from build123d import *

# Parameters (mm, degrees)
SKETCH1_R           = 4
SKETCH1_R_2         = 2
BOSS_EXTRUDE1_DEPTH = 5.4
SKETCH2_R           = 7.5
SKETCH2_R_2         = 4
BOSS_EXTRUDE2_DEPTH = 19


with BuildPart() as part:
    # Sketch1 → Boss-Extrude1 (new body)
    with BuildSketch(Plane(origin=(0, 0, 0), x_dir=(0, 0, -1), z_dir=(1, 0, 0))):
        Polygon((-12.5, 10), (-10, 12.5), (10, 12.5), (12.5, 10), (12.5, -10), (10, -12.5), (-10, -12.5), (-12.5, -10), align=None)
        with Locations(Location((0, 0, 0), (0, 0, 180))):
            Circle(SKETCH1_R, mode=Mode.SUBTRACT)
        with Locations(Location((8.485281374, 8.485281374, 0), (0, 0, 180))):
            Circle(SKETCH1_R_2, mode=Mode.SUBTRACT)
        with Locations(Location((8.485281374, -8.485281374, 0), (0, 0, 180))):
            Circle(SKETCH1_R_2, mode=Mode.SUBTRACT)
        with Locations(Location((-8.485281374, -8.485281374, 0), (0, 0, 180))):
            Circle(SKETCH1_R_2, mode=Mode.SUBTRACT)
        with Locations(Location((-8.485281374, 8.485281374, 0), (0, 0, 180))):
            Circle(SKETCH1_R_2, mode=Mode.SUBTRACT)
    extrude(amount=BOSS_EXTRUDE1_DEPTH)

    # Sketch2 → Boss-Extrude2 (add)
    with BuildSketch(Plane(origin=(5.4, 0, 0), x_dir=(0, 0, -1), z_dir=(1, 0, 0))):
        with Locations(Location((0, 0, 0), (0, 0, 180))):
            Circle(SKETCH2_R)
        with Locations(Location((0, 0, 0), (0, 0, 180))):
            Circle(SKETCH2_R_2, mode=Mode.SUBTRACT)
    extrude(amount=BOSS_EXTRUDE2_DEPTH)


solid = part.part
Geometry: final body of the model. Coordinates: model frame, mm. A direction names the side the tool comes from. Round coordinates to 2 decimals unless told otherwise and drop trailing zeros. Loops run counter-clockwise (first coordinate to the right, second up) from the corner with the lowest first, then second, coordinate; pieces in that order, holes last.
Q1. Access query for faces 5 (the flat face through (2.7, 11.3, -11.2)), 6 (the flat face through (5.4, 6, 5)). Directions: +Z, -Z, +X, -X, +Y, -Y. A direction counts if a zero-diameter tool reaches every point of the face in a straight line with its end or side. Return the directions, or none.
Q2. Section C-C on z = 4.5. Return loops of the section in (x, y), plus the area to 3 significant figures.
Q3. Pull-direction query (Y, two-part tool) for faces 1 (the cylindrical face through (2.662, 9.702, 6.898)), 2 (the cylindrical face through (2.662, -6.533, 8.052)), 3 (the flat face through (3, -12.5, 0)), 4 (the flat face through (3, 0, 12.5)); classes: released by +Y, released by -Y, zero draft, split by the parting line, or undercut.
Q4. Section D-D on x = 4.5. Return loops of the section in (y, z), plus the area to 3 significant figures.
Q5. Material intervals for L1, parallel to Y at x = 17.75, z = 0; L2, parallel to X at y = -9, z = -1.25; L3, parallel to Y at x = 12.5, z = -2.25, sorted ascending.
Q6. Section A-A on z = 0. Return loops of the section in (x, y), plus the area to 3 significant figures.
Q7. Pin query (flat end, axial travel): P1, Ø3.5, axis at y = -8.49, z = -8.49, coming from the -X side; P2, Ø4.5, axis at y = 8.49, z = 8.49, coming from the +X side; P3, Ø5, axis at x = 5.5, y = -8, coming from the +Z side; P4, Ø1.5, axis at x = 10, z = 5, coming from the -Y side. Return the tip coordinate at first contact, or that it passes through.
Evaluation:
1. face 5: -Z, +X, -X, +Y
1. face 6: +X
2. outline: (0, -12.5) - (5.4, -12.5) - (5.4, -6) - (24.4, -6) - (24.4, 6) - (5.4, 6) - (5.4, 12.5) - (0, 12.5) - close
2. area: 363 mm2
3. face 1: undercut
3. face 2: undercut
3. face 3: released by -Y
3. face 4: zero draft
4. outline: (-12.5, -10) - (-10, -12.5) - (10, -12.5) - (12.5, -10) - (12.5, 10) - (10, 12.5) - (-10, 12.5) - (-12.5, 10) - close; hole circle Ø4 at (-8.49, -8.49); hole circle Ø4 at (-8.49, 8.49); hole circle Ø8 at (0, 0); hole circle Ø4 at (8.49, -8.49); hole circle Ø4 at (8.49, 8.49)
4. area: 512 mm2
5. L1: y = -7.5 to -4, 4 to 7.5
5. L2: x = 0 to 5.4
5. L3: y = -7.15 to -3.31, 3.31 to 7.15
6. outline: (0, -12.5) - (5.4, -12.5) - (5.4, -7.5) - (24.4, -7.5) - (24.4, -4) - (0, -4) - close; (0, 4) - (24.4, 4) - (24.4, 7.5) - (5.4, 7.5) - (5.4, 12.5) - (0, 12.5) - close
6. area: 225 mm2
7. P1: passes through
7. P2: stops at x = 5.4
7. P3: stops at z = 12.5
7. P4: stops at y = -6.18
